Model file for the job. Use its own axes, mm. A direction names the side the tool comes from. Coordinates: 2 decimals unless noted, no trailing zeros. Loops run counter-clockwise (first coordinate to the right, second up) from the corner with the lowest first, then second, coordinate; pieces in that order, holes last.
from build123d import *

# Parameters (mm, degrees)
SKETCH1_W             = 7.5
SKETCH1_H             = 22
SKETCH1_R             = 1.5
BOSS_EXTRUDE2_DEPTH   = 27.5
BOSS_EXTRUDE2_2_DEPTH = 27.5
SKETCH1_5_R           = 60
BOSS_EXTRUDE3_DEPTH   = 41
SKETCH1_7_W           = 7.5
SKETCH1_7_H           = 22
SKETCH1_7_R           = 1.5
CUT_EXTRUDE1_DEPTH    = 15
SKETCH2_W             = 56.358839631
SKETCH2_H             = 22
CUT_EXTRUDE2_DEPTH    = 15


with BuildPart() as part:
    # Sketch1 → Boss-Extrude2 (new body)
    with BuildSketch(Plane(origin=(0, 0, 0), x_dir=(1, 0, 0), z_dir=(0, 1, 0))):
        with Locations((-24.75, 0)):
            Rectangle(SKETCH1_W, SKETCH1_H)
        with Locations(Location((-24, -5, 0), (0, 0, 270))):
            Circle(SKETCH1_R, mode=Mode.SUBTRACT)
        with Locations(Location((-24, 5, 0), (0, 0, 270))):
            Circle(SKETCH1_R, mode=Mode.SUBTRACT)
    extrude(amount=BOSS_EXTRUDE2_DEPTH)



with BuildPart() as body_2:
    # Sketch1 → Boss-Extrude2 2 (new body)
    with BuildSketch(Plane(origin=(0, 0, 0), x_dir=(1, 0, 0), z_dir=(0, 1, 0))):
        with Locations((24.75, 0)):
            Rectangle(SKETCH1_W, SKETCH1_H)
        with Locations(Location((24, -5, 0), (0, 0, 270))):
            Circle(SKETCH1_R, mode=Mode.SUBTRACT)
        with Locations(Location((24, 5, 0), (0, 0, 270))):
            Circle(SKETCH1_R, mode=Mode.SUBTRACT)
    extrude(amount=BOSS_EXTRUDE2_2_DEPTH)


with BuildPart() as part_1:
    add(part.part)

    add(body_2.part)  # Boss-Extrude3 merges body 2
    # Sketch1_5 → Boss-Extrude3 (add)
    with BuildSketch(Plane(origin=(0, 0, 0), x_dir=(1, 0, 0), z_dir=(0, 1, 0))):
        with Locations(Location((-11.17, 0, 0), (0, 0, 270))):
            Circle(SKETCH1_5_R)
        Polygon((28.5, -11), (21, -11), (-21, -11), (-28.5, -11), (-28.5, 11), (-21, 11), (21, 11), (28.5, 11), align=None, mode=Mode.SUBTRACT)
    extrude(amount=BOSS_EXTRUDE3_DEPTH)

    # Sketch1_7 → Cut-Extrude1 (cut)
    # profile 1 of 2: a face of its own
    with BuildSketch(Plane(origin=(0, 0, 0), x_dir=(1, 0, 0), z_dir=(0, 1, 0))):
        with Locations((24.75, 0)):
            Rectangle(SKETCH1_7_W, SKETCH1_7_H)
        with Locations(Location((24, -5, 0), (0, 0, 270))):
            Circle(SKETCH1_7_R, mode=Mode.SUBTRACT)
        with Locations(Location((24, 5, 0), (0, 0, 270))):
            Circle(SKETCH1_7_R, mode=Mode.SUBTRACT)
    # profile 2 of 2: a face of its own
    with BuildSketch(Plane(origin=(0, 0, 0), x_dir=(1, 0, 0), z_dir=(0, 1, 0))):
        with Locations((-24.75, 0)):
            Rectangle(SKETCH1_7_W, SKETCH1_7_H)
        with Locations(Location((-24, -5, 0), (0, 0, 270))):
            Circle(SKETCH1_7_R, mode=Mode.SUBTRACT)
        with Locations(Location((-24, 5, 0), (0, 0, 270))):
            Circle(SKETCH1_7_R, mode=Mode.SUBTRACT)
    extrude(amount=CUT_EXTRUDE1_DEPTH, mode=Mode.SUBTRACT)

    # Sketch2 → Cut-Extrude2 (cut)
    with BuildSketch(Plane.XZ):
        with Locations((-56.679419816, 0)):
            Rectangle(SKETCH2_W, SKETCH2_H)
    extrude(amount=-CUT_EXTRUDE2_DEPTH, mode=Mode.SUBTRACT)


solid = part_1.part
Q1. Drill centre lines: line 1 (X direction, y = 21.5, z = 5); line 2 (Z direction, x = -1, y = 9); line 3 (X direction, y = 23, z = -3). Where is each one in solid material? Low to high.
Answers:
line 1: x = -70.96 to -25.5, -22.5 to -21, 21 to 22.5, 25.5 to 48.62
line 2: z = -59.13 to -11, 11 to 59.13
line 3: x = -71.09 to -21, 21 to 48.75
Q2. Slice it at D-D (y = 37). List the corners of the cut face in (x, z).
Answers:
outline: circle Ø120 at (-11.17, 0); hole (-28.5, -11) - (28.5, -11) - (28.5, 11) - (-28.5, 11) - close
Q3. Slice it at B-B (x = -11.17). List the corners of the cut face in (y, z), and give its area (3 significant figures).
Answers:
outline: (0, -60) - (41, -60) - (41, -11) - (0, -11) - close; (0, 11) - (41, 11) - (41, 60) - (0, 60) - close
area: 4,020 mm2
Q4. Which spindle directions (+Z, -Z, +X, -X, +Y, -Y) get a long thin tool onto all of the face, cutting with end or side? Do faces 4 (the flat face through (-21, 21, 0)), 5 (the flat face through (28.5, 34, 0)), 6 (the flat face through (25, 15, 0)). Say none if no direction does.
Answers:
face 4: +Y, -Y
face 5: +Y
face 6: -X, -Y
Q5. Slice it at A-A (z = 0). List the corners of the cut face in (x, y), and give its area (3 significant figures).
Answers:
outline: (-71.17, 15) - (-21, 15) - (-21, 27.5) - (-28.5, 27.5) - (-28.5, 41) - (-71.17, 41) - close; (21, 15) - (28.5, 15) - (28.5, 0) - (48.83, 0) - (48.83, 41) - (28.5, 41) - (28.5, 27.5) - (21, 27.5) - close
area: 2,130 mm2
Q6. Flat gauge pins, fed straight in: P1, Ø3, axis at y = 19, z = 47.5, coming from the +X side; P2, Ø12.5, axis at x = -12, y = 23.5, coming from the -Z side; P3, Ø1, axis at y = 9.5, z = 33, coming from the -X side; P4, Ø3.5, axis at x = 24, z = 5, coming from the +Y side. Where does each tip first touch, or does it go through?
Answers:
P1: stops at x = 27.35
P2: stops at z = -60
P3: stops at x = -61.61
P4: stops at y = 27.5
Q7. Slice it at C-C (y = 21.5). List the corners of the cut face in (x, z), and give its area (3 significant figures).
Answers:
outline: circle Ø120 at (-11.17, 0); hole circle Ø3 at (-24, -5); hole circle Ø3 at (-24, 5); hole (-21, -11) - (21, -11) - (21, 11) - (-21, 11) - close; hole circle Ø3 at (24, -5); hole circle Ø3 at (24, 5)
area: 10,400 mm2
Q8. Mould opens along X. For faces 1 (the flat face through (-46, 15, 0)), 2 (the cylindrical face through (-22.735, 21.162, 5.806)), 3 (the cylindrical face through (-69.743, 20.213, -13.007)) say: +X half, -X half, draft (parallel to the pull), parting line (faces both ways), or undercut.
Answers:
face 1: draft
face 2: undercut
face 3: parting line
